Check sheet for the modelled part. Datum: model origin and axes. Units: mm. A direction names the side the tool comes from. Round coordinates to 2 decimals unless told otherwise and drop trailing zeros. Order: outer loops, then holes, each group sorted by start corner. A loop starts at its lowest first (then second) coordinate and runs counter-clockwise, first axis right, second up. Notation, with made-up numbers: (30, 28.5) -> (38, 28.5) arc R17 cw to (38, 40.5) -> close; hole circle Ø3 at (0, 12.25). An arc over 180 degrees is marked (long way). Answer as CSV lines item,"result". Start each with the question number.
from build123d import *

# Parameters (mm, degrees)
F0_W     = 18.975
F0_H     = 33
F0_W_2   = 20.5
F1_DEPTH = 27
F2_W     = 13
F2_H     = 13
F3_DEPTH = 27.001
F4_W     = 1.5
F4_H     = 13
F5_DEPTH = 4.25


with BuildPart() as f1:
    # F0 (on Top) → F1 (new body)
    with BuildSketch(Plane.XY):
        with Locations((19.7375, 0)):
            Rectangle(F0_W, F0_H)
        Rectangle(F0_W_2, F0_H)
        with Locations((-19.7375, 0)):
            Rectangle(F0_W, F0_H)
    extrude(amount=F1_DEPTH)

    # F2 (on face) → F3 (cut, through all)
    with BuildSketch(Plane.XY):
        with Locations((0, 10)):
            Rectangle(F2_W, F2_H)
    extrude(amount=F3_DEPTH, mode=Mode.SUBTRACT)

    # F4 (on face) → F5 (join)
    with BuildSketch(Plane.XY):
        with Locations((-5.75, 10)):
            Rectangle(F4_W, F4_H)
        with Locations((5.75, 10)):
            Rectangle(F4_W, F4_H)
    extrude(amount=F5_DEPTH)


solid = f1.part
1) Mould release check, pull along X, two halves, no side actions. Record for faces 1 (the face through (0, 3.5, 13)), 2 (the face through (29.225, 0, 13)), 3 (the face through (-29.225, 0, 13)), 4 (the face through (0, 0, 0)): released by +X, released by -X, zero draft, split by the parting line, or undercut.
2) Material ranges on line 1 along X through (y, z) = (11, 18) (3 decimals); line 2 along Y through (x, z) = (-2, 17), recorded low to high.
3) Depth check by flat-ended pin: pin 1 Ø3 at (x, y) = (4.5, 10) entering from +Z. Enter the tip coordinate at first touch or a pass-through.
4) Section check A-A on y = 13. Record the cut outline in (x, z) (3 decimals).
5) Access from +Z, -Z, +X, -X, +Y, -Y to the whole of each face (thin tool, end or side, straight path). Record for faces 5 (the face through (6, 10, 4.25)), 6 (the face through (5, 10, 2)), 7 (the face through (0, 0, 27)).
6) Section check B-B on z = 14. Record the cut outline in (x, y) (3 decimals).
Solutions:
1,face 1,"undercut"
1,face 2,"released by +X"
1,face 3,"released by -X"
1,face 4,"zero draft"
2,line 1,"x = -29.225 to -6.5, 6.5 to 29.225"
2,line 2,"y = -16.5 to 3.5"
3,pin 1,"stops at z = 4.25"
4,outline,"(-29.225, 0) -> (-5, 0) -> (-5, 4.25) -> (-6.5, 4.25) -> (-6.5, 27) -> (-29.225, 27) -> close; (5, 0) -> (29.225, 0) -> (29.225, 27) -> (6.5, 27) -> (6.5, 4.25) -> (5, 4.25) -> close"
5,face 5,"+Z, +Y"
5,face 6,"+Z, -Z, +Y"
5,face 7,"+Z, +X, -X, +Y, -Y"
6,outline,"(-29.225, -16.5) -> (29.225, -16.5) -> (29.225, 16.5) -> (6.5, 16.5) -> (6.5, 3.5) -> (-6.5, 3.5) -> (-6.5, 16.5) -> (-29.225, 16.5) -> close"
